Can you work these out from the model? Positions are in its coordinate system, mm. A direction names the side the tool comes from. Coordinates: 2 decimals unless noted, no trailing zeros. Order: outer loops, then holes, each group sorted by start corner. A loop starts at its lowest first (then second) coordinate and runs counter-clockwise, first axis right, second up. Notation, with made-up numbers: (25, -29) -> (72, -29) arc R13 cw to (72, -25) -> close; hole circle Ø2 at (65, 73). An arc over 180 degrees is marked (long way). Answer in a Markdown table with one row per item. Add a question column.
1. On a 3-axis mill with a long thin cutter (end or side, diameter ignored), from which of +Z, -Z, +X, -X, +Y, -Y can I reach the whole of each face in a straight line? I mean faces 4 (the face through (50.09, -22.76, 0.14)), 5 (the face through (53, -9.828, -3)), 6 (the face through (55, 18.112, 0)). Say none if no direction works.
2. Imagine slicing it at A-A on y = 13.5. Write out the boundary of the cut face in (x, z).
3. Will these pins go through, and if not, where does the flat tip stop? pin 1 (2 mm diameter, centred on x = 49, z = -7.5, fed in from -Y); pin 2 (11 mm diameter, centred on x = 51.5, z = 3, fed in from +Y); pin 3 (2 mm diameter, centred on y = -18, z = 0, fed in from -X); pin 4 (5 mm diameter, centred on x = 49.47, z = 0, fed in from +Y).
4. We'd pull the mould along X, two halves only. Please class faces 1 (the face through (44.65, -5.13, -3.07)), 2 (the face through (44, 47.322, -5)), 3 (the face through (52, -7.288, 0)): pulls with the +X half, pulls with the -X half, needs draft (parallel to the pull), parting line crosses it, or undercut.
5. Imagine slicing it at B-B on y = 37. Write out the boundary of the cut face in (x, z) (3 decimals), plus the area to 3 significant figures.
6. If I drill on line 1 along X through (y, z) = (25, 0); line 2 along X through (y, z) = (6.25, 0); line 3 along Z through (x, y) = (46, 4), over which ranges is the centre line in solid material (lowest first)? Write a range as [from, to].
from build123d import *

# Parameters (mm, degrees)
SKETCH1_W = 3.175
SKETCH1_H = 9.525
SHELL1_T  = -2.54


with BuildPart() as part:
    # Sketch1 → Revolve5 (revolve)
    with BuildSketch(Plane.XY, mode=Mode.PRIVATE) as revolve5_sk:
        Polygon((49.470878753, 15.571822686), (49.470878753, 47.321822686), (39.945878753, 47.321822686), (39.945878753, 15.571822686), (41.850878753, 15.571822686), align=None)
        Polygon((49.470878753, 9.221822686), (49.470878753, 15.571822686), (41.850878753, 15.571822686), (41.850878753, 9.221822686), (43.120878753, 9.221822686), align=None)
        Polygon((49.470878753, -0.303177314), (49.470878753, 9.221822686), (43.120878753, 9.221822686), (43.120878753, -0.303177314), (43.755878753, -0.303177314), align=None)
        Polygon((49.470878753, -9.828177314), (49.470878753, -0.303177314), (43.755878753, -0.303177314), (43.755878753, -9.828177314), (45.025878753, -9.828177314), align=None)
        Polygon((49.470878753, -19.353177314), (49.470878753, -9.828177314), (45.025878753, -9.828177314), (45.025878753, -19.353177314), (46.295878753, -19.353177314), align=None)
        with Locations((47.883378753, -24.115677314)):
            Rectangle(SKETCH1_W, SKETCH1_H)
    revolve(revolve5_sk.sketch.rotate(Axis((49.470878753, -38.227970454, 0), (0, 1, 0)), 270), axis=Axis((49.470878753, -38.227970454, 0), (0, 1, 0)))

    # Shell1
    shell1_openings = [part.faces().sort_by_distance(p)[0] for p in [
        (49.470878753, 47.321822686, 0),
        (49.470878753, -28.878177314, 0),
    ]]
    offset(amount=SHELL1_T, openings=shell1_openings, kind=Kind.INTERSECTION)


solid = part.part
Answers follow:
| question | item | result |
|---|---|---|
| 1 | face 4 | +Y, -Y |
| 1 | face 5 | -Y |
| 1 | face 6 | +Y |
| 2 | outline | circle Ø15.24 at (49.47, 0); hole circle Ø10.16 at (49.47, 0) |
| 3 | pin 1 | stops at y = 9.22 |
| 3 | pin 2 | stops at y = 47.32 |
| 3 | pin 3 | stops at x = 45.03 |
| 3 | pin 4 | stops at y = -7.29 |
| 4 | face 1 | parting line crosses it |
| 4 | face 2 | needs draft |
| 4 | face 3 | undercut |
| 5 | outline | circle Ø19.05 at (49.471, 0); hole circle Ø13.97 at (49.471, 0) |
| 5 | area | 132 mm² |
| 6 | line 1 | x = [39.95, 42.49], [56.46, 59] |
| 6 | line 2 | x = [43.12, 45.66], [53.28, 55.82] |
| 6 | line 3 | z = [-5.32, -1.57], [1.57, 5.32] |
